Input: part model. Units: mm. Frame: model coordinates. A direction names the side the tool comes from. Give positions to 0.01 mm unless a question says otherwise; leave off trailing zeros. Loops run counter-clockwise (first coordinate to the right, second up) from the corner with the lowest first, then second, coordinate; pieces in that order, holes last. Notation, with made-up numbers: M -10.5,84 L -3.5,84 A27 cw -3.5,105 Z; hole C 50,35 d6. An arc over 180 degrees is marked long. Answer as a JSON object with one key per item and string values. Group by question number.
```python
from build123d import *

# Parameters (mm, degrees)
F0_R     = 1.5
F1_DEPTH = 3


with BuildPart() as f1:
    # F0 (on Top) → F1 (new body)
    with BuildSketch(Plane.XY):
        with BuildLine():
            Line((-25, 10), (-30, 10))
            Line((-30, 10), (-30, -5.5))
            Line((-30, -5.5), (30, -5.5))
            Line((30, -5.5), (30, 10))
            Line((30, 10), (25, 10))
            Line((25, 10), (25, 5))
            Line((25, 5), (22, 5))
            Line((22, 5), (22, 10))
            Line((22, 10), (17, 10))
            Line((17, 10), (17, 4))
            ThreePointArc((17, 4), (16.56066, 2.93934), (15.5, 2.5))
            Line((15.5, 2.5), (-15.5, 2.5))
            ThreePointArc((-15.5, 2.5), (-16.56066, 2.93934), (-17, 4))
            Line((-17, 4), (-17, 10))
            Line((-17, 10), (-22, 10))
            Line((-22, 10), (-22, 5))
            Line((-22, 5), (-25, 5))
            Line((-25, 5), (-25, 10))
        make_face()
        with Locations((-23.5, 0)):
            Circle(F0_R, mode=Mode.SUBTRACT)
        with Locations((-13, -1.5)):
            Circle(F0_R, mode=Mode.SUBTRACT)
        with Locations((0, -1.5)):
            Circle(F0_R, mode=Mode.SUBTRACT)
        with Locations((13, -1.5)):
            Circle(F0_R, mode=Mode.SUBTRACT)
        with Locations((23.5, 0)):
            Circle(F0_R, mode=Mode.SUBTRACT)
    extrude(amount=F1_DEPTH)


solid = f1.part
```
1. Material intervals for L1, parallel to Y at x = 0, z = 2.1; L2, parallel to X at y = 9.25, z = 1.15; L3, parallel to X at y = 4, z = 1.6, sorted ascending.
2. Reachability of faces 1 (the cylindrical face through (0, -3, 1)), 2 (the flat face through (24, 5, 1)) from +Z, -Z, +X, -X, +Y, -Y: full face, straight path, thin tool, end or side. Return the list, or none.
3. Section B-B (y = 6.75). Output: boundary loops of the cut face in (x, z), then the cut area to 3 significant figures.
4. Section C-C (z = 2.3). Output: boundary loops of the cut face in (x, y).
5. Section A-A (x = -23.5). Output: boundary loops of the cut face in (y, z).
6. Section D-D (y = 0.5). Output: boundary loops of the cut face in (x, z).
7. First-contact query: P1, Ø0.9, axis at x = 24, z = 2, coming from the +Y side. Flat tip, straight axial feed; report the tip coordinate or a pass-through.
8. Mould query, pull axis X, two halves, no side actions, for faces 3 (the flat face through (0, 1, 0)), 4 (the cylindrical face through (22, 0, 1)), 5 (the flat face through (30, 2, 1)). Classes: pulls with the +X half, pulls with the -X half, needs draft (parallel to the pull), parting line crosses it, or undercut.
Geometry results:
{
 "1": {"L1": "-5.5 to -3, 0 to 2.5", "L2": "-30 to -25, -22 to -17, 17 to 22, 25 to 30", "L3": "-30 to -17, 17 to 30"},
 "2": {"face 1": "+Z, -Z", "face 2": "+Z, -Z, +Y"},
 "3": {"outline": "M -30,0 L -25,0 L -25,3 L -30,3 Z; M -22,0 L -17,0 L -17,3 L -22,3 Z; M 17,0 L 22,0 L 22,3 L 17,3 Z; M 25,0 L 30,0 L 30,3 L 25,3 Z", "area": "60.0 mm2"},
 "4": {"outline": "M -30,-5.5 L 30,-5.5 L 30,10 L 25,10 L 25,5 L 22,5 L 22,10 L 17,10 L 17,4 A1.5 cw 15.5,2.5 L -15.5,2.5 A1.5 cw -17,4 L -17,10 L -22,10 L -22,5 L -25,5 L -25,10 L -30,10 Z; hole C -23.5,0 d3; hole C -13,-1.5 d3; hole C 0,-1.5 d3; hole C 13,-1.5 d3; hole C 23.5,0 d3"},
 "5": {"outline": "M -5.5,0 L -1.5,0 L -1.5,3 L -5.5,3 Z; M 1.5,0 L 5,0 L 5,3 L 1.5,3 Z"},
 "6": {"outline": "M -30,0 L -24.91,0 L -24.91,3 L -30,3 Z; M -22.09,0 L 22.09,0 L 22.09,3 L -22.09,3 Z; M 24.91,0 L 30,0 L 30,3 L 24.91,3 Z"},
 "7": {"P1": "y = 5"},
 "8": {"face 3": "needs draft", "face 4": "undercut", "face 5": "pulls with the +X half"}
}
